Could you check a few things on this model? Use its own coordinates, in mm. Face numbers are marked on the shaded views. Round coordinates to 2 decimals unless told otherwise and drop trailing zeros. Write each loop counter-clockwise with the first axis right and the second up, starting at its lowest first coordinate (ties: lowest second). Pieces come first, ordered by that corner, then holes. Notation, with made-up numbers: (56.5, -34) -> (85.5, -34) arc R28 ccw to (85.5, -4) -> close; hole circle Ø11 at (-25, -10.5). An arc over 180 degrees is marked (long way). Answer as CSV lines item,"result". Start each with the question number.
Q1. Imagine slicing it at B-B on z = 0. Please give me the cut outline in (x, y).
Q2. If I drill on line 1 (Z direction, x = 1, y = 14.75); line 2 (X direction, y = 10.25, z = 0); line 3 (X direction, y = 13.5, z = -16.5), over which ranges is the centre line in solid material (lowest first)? Write a range as [from, to].
Q3. Imagine slicing it at C-C on y = 4.5. Please give me the cut outline in (x, z).
Q4. Will these pins go through, and if not, where does the flat tip stop? pin 1 Ø5 at (x, y) = (8.5, 13) entering from -Z; pin 2 Ø12 at (x, y) = (-15, 6) entering from +Z.
Q5. If we mould it in two halves opening along Z, with no side actions, what happens to the marked faces 1 and 2? For each: pulls with the +Z half, pulls with the -Z half, needs draft (parallel to the pull), parting line crosses it, or undercut.
Q6. Imagine slicing it at A-A on x = 0. Please give me the cut outline in (y, z).
Q7. Imagine slicing it at D-D on y = 9.75. Please give me the cut outline in (x, z).
from build123d import *

# Parameters (mm, degrees)
SKETCH1_R           = 50.8
SKETCH1_R_2         = 49.53
BOSS_EXTRUDE1_DEPTH = 25.4
SKETCH2_R           = 2.38125
CUT_EXTRUDE1_DEPTH  = 25.4
SKETCH3_R           = 1.5875
CUT_EXTRUDE2_DEPTH  = 37.338
CIRPATTERN1_COUNT   = 4


with BuildPart() as part:
    # Sketch1 → Boss-Extrude1 (new body)
    with BuildSketch(Plane(origin=(0, 0, 0), x_dir=(1, 0, 0), z_dir=(0, 1, 0))):
        Circle(SKETCH1_R)
        Circle(SKETCH1_R_2, mode=Mode.SUBTRACT)
    extrude(amount=BOSS_EXTRUDE1_DEPTH)

    # Sketch2 → Cut-Extrude1 (cut)
    with BuildSketch(Plane(origin=(80.709285485, 206.333156205, 111.645979585), x_dir=(0, -1, 0), z_dir=(0.969338628, 0, -0.24572876))):
        with Locations((196.808156205, 128.055353348)):
            Circle(SKETCH2_R)
        with Locations((190.458156205, 128.055353348)):
            Circle(SKETCH2_R)
    extrude(amount=-CUT_EXTRUDE1_DEPTH, mode=Mode.SUBTRACT)

    # Sketch3 → Cut-Extrude2 (cut)
    with BuildSketch(Plane(origin=(-3.10026152, 207.778194099, 134.798971935), x_dir=(0, 1, 0), z_dir=(-0.962336257, 0, -0.271861966))):
        with Locations((-195.078194099, 130.56478129)):
            Circle(SKETCH3_R)
    cut_extrude2 = extrude(amount=-CUT_EXTRUDE2_DEPTH, mode=Mode.SUBTRACT)

    # CirPattern1: Cut-Extrude2 ×4 about axis
    cirpattern1_axis = Axis((0, 0, 0), (0, -1, 0))
    for i in range(1, CIRPATTERN1_COUNT):
        add(cut_extrude2.rotate(cirpattern1_axis, i * 360 / CIRPATTERN1_COUNT), mode=Mode.SUBTRACT)


solid = part.part
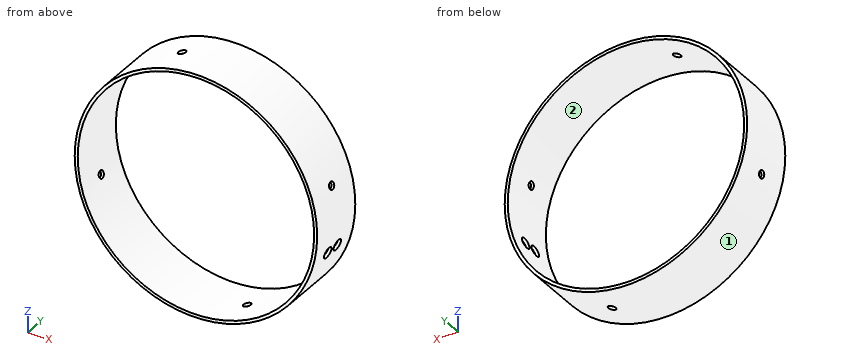
Checks:
1,outline,"(-50.8, 0) -> (-49.53, 0) -> (-49.53, 25.4) -> (-50.8, 25.4) -> close; (49.53, 0) -> (50.8, 0) -> (50.8, 25.4) -> (49.53, 25.4) -> close"
2,line 1,"[-50.79, -49.52], [49.52, 50.79]"
2,line 2,"[-50.8, -49.53], [49.53, 50.8]"
2,line 3,"[-48.05, -46.7], [46.7, 48.05]"
3,outline,"circle Ø101.6 at (0, 0); hole circle Ø99.06 at (0, 0)"
4,pin 1,"z = -50.44"
4,pin 2,"z = 50"
5,face 1,"parting line crosses it"
5,face 2,"undercut"
6,outline,"(0, -50.8) -> (25.4, -50.8) -> (25.4, -49.53) -> (0, -49.53) -> close; (0, 49.53) -> (25.4, 49.53) -> (25.4, 50.8) -> (0, 50.8) -> close"
7,outline,"(47.37, -14.45) arc R49.53 cw (long way) to (48.54, -9.86) -> (49.77, -10.17) arc R50.8 ccw (long way) to (48.61, -14.77) -> close"
